from build123d import *

# Parameters (mm, degrees)
EXTRUDE_1_DEPTH     = 13
SKETCH_4_R          = 3.5
CUT_EXTRUDE_3_DEPTH = 40.419530037
SKETCH_5_R          = 1.1
CUT_EXTRUDE_4_DEPTH = 10


with BuildPart() as part:
    # 草图1 → 凸台-拉伸1 (new body)
    with BuildSketch(Plane(origin=(0, 0, 0), x_dir=(1, 0, 0), z_dir=(0, 1, 0))):
        with BuildLine():
            Line((0, 35), (6.5, 35))
            Line((6.5, 35), (5.5, 20))
            Line((5.5, 20), (10.30634728, 20))
            add(Edge.make_bspline(
                [(10.30634728, 20), (13.762117506, 18.48353704), (16, 15.5)],
                knots=[0, 0, 0, 1, 1, 1], degree=2))
            Line((16, 15.5), (16, 15))
            Line((16, 15), (5.5, 15))
            Line((5.5, 15), (5.5, 0))
            Line((5.5, 0), (0, 0))
            Line((0, 0), (0.3, 0.3))
            Line((0.3, 0.3), (0, 0.6))
            Line((0, 0.6), (0.3, 0.9))
            Line((0.3, 0.9), (0, 1.2))
            Line((0, 1.2), (0.3, 1.5))
            Line((0.3, 1.5), (0, 1.8))
            Line((0, 1.8), (0.3, 2.1))
            Line((0.3, 2.1), (0, 2.4))
            Line((0, 2.4), (0.3, 2.7))
            Line((0.3, 2.7), (0, 3))
            Line((0, 3), (0.3, 3.3))
            Line((0.3, 3.3), (0, 3.6))
            Line((0, 3.6), (0.3, 3.9))
            Line((0.3, 3.9), (0, 4.2))
            Line((0, 4.2), (0.3, 4.5))
            Line((0.3, 4.5), (0, 4.8))
            Line((0, 4.8), (0.3, 5.1))
            Line((0.3, 5.1), (0, 5.4))
            Line((0, 5.4), (0.3, 5.7))
            Line((0.3, 5.7), (0, 6))
            Line((0, 6), (0.3, 6.3))
            Line((0.3, 6.3), (0, 6.6))
            Line((0, 6.6), (0.3, 6.9))
            Line((0.3, 6.9), (0, 7.2))
            Line((0, 7.2), (0.3, 7.5))
            Line((0.3, 7.5), (0, 7.8))
            Line((0, 7.8), (0.3, 8.1))
            Line((0.3, 8.1), (0, 8.4))
            Line((0, 8.4), (0.3, 8.7))
            Line((0.3, 8.7), (0, 9))
            Line((0, 9), (0.3, 9.3))
            Line((0.3, 9.3), (0, 9.6))
            Line((0, 9.6), (0.3, 9.9))
            Line((0.3, 9.9), (0, 10.2))
            Line((0, 10.2), (0.3, 10.5))
            Line((0.3, 10.5), (0, 10.8))
            Line((0, 10.8), (0.3, 11.1))
            Line((0.3, 11.1), (0, 11.4))
            Line((0, 11.4), (0.3, 11.7))
            Line((0.3, 11.7), (0, 12))
            Line((0, 12), (0.3, 12.3))
            Line((0.3, 12.3), (0, 12.6))
            Line((0, 12.6), (0.3, 12.9))
            Line((0.3, 12.9), (0, 13.2))
            Line((0, 13.2), (0.3, 13.5))
            Line((0.3, 13.5), (0, 13.8))
            Line((0, 13.8), (0.3, 14.1))
            Line((0.3, 14.1), (0, 14.4))
            Line((0, 14.4), (0.3, 14.7))
            Line((0.3, 14.7), (0, 15))
            Line((0, 15), (0.3, 15.3))
            Line((0.3, 15.3), (0, 15.6))
            Line((0, 15.6), (0.3, 15.9))
            Line((0.3, 15.9), (0, 16.2))
            Line((0, 16.2), (0.3, 16.5))
            Line((0.3, 16.5), (0, 16.8))
            Line((0, 16.8), (0.3, 17.1))
            Line((0.3, 17.1), (0, 17.4))
            Line((0, 17.4), (0.3, 17.7))
            Line((0.3, 17.7), (0, 18))
            Line((0, 18), (0.3, 18.3))
            Line((0.3, 18.3), (0, 18.6))
            Line((0, 18.6), (0.3, 18.9))
            Line((0.3, 18.9), (0, 19.2))
            Line((0, 19.2), (0.3, 19.5))
            Line((0.3, 19.5), (0, 19.8))
            Line((0, 19.8), (0.3, 20.1))
            Line((0.3, 20.1), (0, 20.4))
            Line((0, 20.4), (0.3, 20.7))
            Line((0.3, 20.7), (0, 21))
            Line((0, 21), (0.3, 21.3))
            Line((0.3, 21.3), (0, 21.6))
            Line((0, 21.6), (0.3, 21.9))
            Line((0.3, 21.9), (0, 22.2))
            Line((0, 22.2), (0.3, 22.5))
            Line((0.3, 22.5), (0, 22.8))
            Line((0, 22.8), (0.3, 23.1))
            Line((0.3, 23.1), (0, 23.4))
            Line((0, 23.4), (0.3, 23.7))
            Line((0.3, 23.7), (0, 24))
            Line((0, 24), (0, 35))
        make_face()
    extrude(amount=EXTRUDE_1_DEPTH)

    # 草图4 → 切除-拉伸3 (cut, through all)
    with BuildSketch(Plane(origin=(4.148230088, 0, 0.276548673), x_dir=(0.06651901052377392, 0, -0.9977851578566089), z_dir=(0.9977851578566089, 0, 0.06651901052377392))):
        with Locations((27.838205904, 7)):
            Circle(SKETCH_4_R)
    extrude(amount=-CUT_EXTRUDE_3_DEPTH, mode=Mode.SUBTRACT)

    # 草图5 → 切除-拉伸4 (cut)
    with BuildSketch(Plane(origin=(5.5, 0, 0), x_dir=(0, 0, -1), z_dir=(1, 0, 0))):
        with Locations((10.8, 6.5)):
            Circle(SKETCH_5_R)
        with Locations((4.3, 6.5)):
            Circle(SKETCH_5_R)
    extrude(amount=-CUT_EXTRUDE_4_DEPTH, mode=Mode.SUBTRACT)


solid = part.part
For this review, take the finished solid that the model builds, in its own axes (mm). A direction names the side the tool comes from. Round coordinates to 2 decimals unless told otherwise and drop trailing zeros. Loops run counter-clockwise (first coordinate to the right, second up) from the corner with the lowest first, then second, coordinate; pieces in that order, holes last. Notation, with made-up numbers: (-14.5, 89) - (35.5, 89) arc R26 ccw to (35.5, 126) - close; hole circle Ø3 at (78.25, 34.25). An arc over 180 degrees is marked (long way). One line per item, written item: value. Start each with the question number.
Item 1: Clearance check with flat-ended pins moving along their axes: pin 1 Ø5 at (x, y) = (13.5, 8) entering from +Z; pin 2 Ø3.5 at (y, z) = (6.5, -10.8) entering from +X; pin 3 Ø5 at (x, y) = (11.5, 5) entering from -Z. State where each tip first meets the part, or that it passes through.
Item 2: The part is to be moulded in two halves that separate along Z. For faces 1 (the flat face through (5, 0, -18)), 2 (the flat face through (6.12, 3.52, -29.27)), 3 (the flat face through (3, 6, 0)), say which applies: +Z half, -Z half, draft (parallel to the pull), parting line (faces both ways), or undercut.
Item 3: Take a section at B-B (x = 5). State how many separate pieces and enclosed holes the cut face has, plus the area to 3 significant figures.
Item 4: For L1, parallel to Z at x = 1.7, y = 6.5; L2, parallel to Y at x = 2.5, z = -10.8; L3, parallel to Z at x = 2.65, y = 6.5, list the stretches that pass through material, from the lowest coordinate up.
Item 5: For faces 4 (the flat face through (0, 6, -32)), 5 (the flat face through (11, 6, -15)), 6 (the flat face through (8, 6, -20)), list the 3-axis set-ups (+Z, -Z, +X, -X, +Y, -Y) from which the entire face can be reached by the end or side of a thin tool; tool diameter is ignored.
Item 6: Take a section at A-A (x = 8.5). Give the boundary of the cut face in (y, z).
Answer below:
1. pin 1: stops at z = -15
1. pin 2: stops at x = 5.5
1. pin 3: stops at z = -20
2. face 1: draft
2. face 2: undercut
2. face 3: +Z half
3. separate pieces: 1
3. enclosed holes: 3
3. area: 409 mm2
4. L1: z = -35 to -31.26, -24.31 to -11.9, -9.7 to -5.4, -3.2 to 0
4. L2: y = 0 to 5.4, 7.6 to 13
4. L3: z = -35 to -31.2, -24.25 to -11.9, -9.7 to -5.4, -3.2 to 0
5. face 4: +Z, -Z, -X, +Y, -Y
5. face 5: +Z, +X, +Y, -Y
5. face 6: +X, +Y, -Y
6. outline: (0, -20) - (13, -20) - (13, -15) - (0, -15) - close
